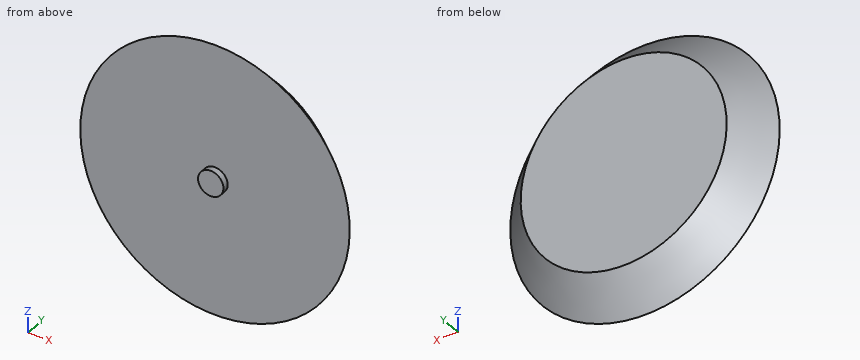
```python
from build123d import *

# Parameters (mm, degrees)
SKETCH1_R           = 8.5
BOSS_EXTRUDE1_DEPTH = 2
CHAMFER1_SIZE       = 2
SKETCH2_R           = 0.8
BOSS_EXTRUDE2_DEPTH = 0.4


with BuildPart() as part:
    # Sketch1 → Boss-Extrude1 (new body)
    with BuildSketch(Plane(origin=(0, 0, 0), x_dir=(1, 0, 0), z_dir=(0, 1, 0))):
        with Locations(Location((0, 0, 0), (0, 0, 270))):
            Circle(SKETCH1_R)
    extrude(amount=BOSS_EXTRUDE1_DEPTH)

    # Chamfer1
    chamfer1_edges = [part.edges().sort_by_distance(p)[0] for p in [
        (0, 2, -8.5),
    ]]
    chamfer(chamfer1_edges, length=CHAMFER1_SIZE - 0.0001)  # a hair under: the kernel refuses the full size

    # Sketch2 → Boss-Extrude2 (add)
    with BuildSketch(Plane(origin=(0, 0, 0), x_dir=(-1, 0, 0), z_dir=(0, -1, 0))):
        with Locations(Location((0, 0, 0), (0, 0, 270))):
            Circle(SKETCH2_R)
    extrude(amount=BOSS_EXTRUDE2_DEPTH)


solid = part.part
```
Geometry check sheet. Reference: the model listing, model coordinates, mm. Coordinates: 2 decimals unless noted, no trailing zeros. Write each loop counter-clockwise with the first axis right and the second up, starting at its lowest first coordinate (ties: lowest second). Pieces come first, ordered by that corner, then holes. Notation, with made-up numbers: M 78,-8 L 122,-8 A23 cw 122,24 Z; hole C 57,-10 d11. An arc over 180 degrees is marked long. Use one line per item in the form item = value. Start each with the question number.
1) Section check C-C on y = 0.75. Enter the section's corners in (x, z), and give its area (3 significant figures).
2) Thickness scan on probe 1 along Y at (x, z) = (0.5, 5.75); probe 2 along Z at (x, y) = (3.5, 1.75); probe 3 along Z at (x, y) = (-3.5, 0.15). Record the ranges inside material, lowest first. Write a range as from..to.
3) Go/stop test with flat-tipped pins: pin 1 Ø1.5 at (x, z) = (3.5, -4.5) entering from -Y; pin 2 Ø1 at (x, y) = (1, 0) entering from +Z. Record where each tip stops, or that it passes through.
Responses:
q1.outline = C 0,0 d15.5
q1.area = 189 mm2
q2.probe_1 = 0..2
q2.probe_2 = -5.77..5.77
q2.probe_3 = -7.58..7.58
q3.pin_1 = 0
q3.pin_2 = 8.49
